```python
from build123d import *

# Parameters (mm, degrees)
ESTRUSIONE_ESTRUSIONE1_DEPTH = 10
RACCORDO1_R                  = 2


with BuildPart() as part:
    # Schizzo1 → Estrusione-Estrusione1 (new body)
    with BuildSketch(Plane.XY):
        with BuildLine():
            Line((-18, 0), (-18, 45.576734941))
            ThreePointArc((-18, 45.576734941), (0.394139103, 39.209366163), (18, 47.511257547))
            Line((18, 47.511257547), (18, 0))
            Line((18, 0), (-18, 0))
        make_face()
    extrude(amount=ESTRUSIONE_ESTRUSIONE1_DEPTH)

    # Raccordo1
    raccordo1_edges = [part.edges().sort_by_distance(p)[0] for p in [
        (-18, 45.576734941, 5),
        (18, 47.511257547, 5),
    ]]
    fillet(raccordo1_edges, radius=RACCORDO1_R)


solid = part.part
```
Build history of the part. All positions in model axes, mm. Coordinates: 2 decimals unless noted, no trailing zeros. Order: outer loops, then holes, each group sorted by start corner. A loop starts at its lowest first (then second) coordinate and runs counter-clockwise, first axis right, second up. Notation, with made-up numbers: M -37,-39.5 L -12,-39.5 A10 cw -12,-22.5 Z; hole C 68,49.5 d11. An arc over 180 degrees is marked long. One line per question, with ' | ' between items. Start each with the question number.
1. Cut at A-A (z = 8). Write the cut outline in (x, y).
2. Cut at C-C (x = -5). Write the cut outline in (y, z).
3. Flat gauge pins, fed straight in: P1, Ø2, axis at x = 11, y = 17, coming from the -Z side; P2, Ø6, axis at x = -14, z = 3.5, coming from the +Y side; P3, Ø1, axis at x = -8, z = 5, coming from the +Y side. Where does each tip first touch, or does it go through?
4. Mould opens along X. For faces 1 (the face through (-16.99, 43.31, 5.07)), 2 (the face through (16.85, 44.78, 5.07)), 3 (the face through (18, 22, 5)), 4 (the face through (0, 23, 0)) say: +X half, -X half, draft (parallel to the pull), parting line (faces both ways), or undercut.
5. Cut at B-B (x = 9). Write the cut outline in (y, z).
6. Wall check: line 1 along Y through (x, z) = (-16, 9.25); line 2 along Y through (x, z) = (-3, 6.5). Give the ranges that are in metal, low to high. Write a range as [from, to].
The answers:
1) outline: M -18,0 L 18,0 L 18,42.97 A2 ccw 14.78,44.55 A25.79 cw -14.92,43.26 A2 ccw -18,41.57 Z
2) outline: M 0,0 L 39.49,0 L 39.49,10 L 0,10 Z
3) P1: stops at z = 0 | P2: stops at y = 43.57 | P3: stops at y = 40.29
4) face 1: undercut | face 2: parting line | face 3: +X half | face 4: draft
5) outline: M 0,0 L 41.19,0 L 41.19,10 L 0,10 Z
6) line 1: y = [0, 43.57] | line 2: y = [0, 39.25]
